Part model, mm, in its own coordinate system. A direction names the side the tool comes from. Give positions to 0.01 mm unless a question says otherwise; leave off trailing zeros. Write each loop counter-clockwise with the first axis right and the second up, starting at its lowest first coordinate (ties: lowest second). Pieces come first, ordered by that corner, then holes. Notation, with made-up numbers: M 23,56 L 70,56 A32 ccw 70,84 Z; hole C 13.25,30.25 d2. An arc over 180 degrees is marked long. Use CSV: the item, a comma, the result in double quotes. Start each with the question number.
1. Band-saw the part on A-A, the plane y = 59.5. List the corners of the cut face in (x, z).
2. Mould opens along Y. For faces 1 (the face through (43, 68, -11.1)), 2 (the face through (30.5, 23, -9)), 3 (the face through (43, 10, -14)) say: pulls with the +Y half, pulls with the -Y half, needs draft (parallel to the pull), parting line crosses it, or undercut.
3. Band-saw the part on B-B, the plane z = -14. Count the separate pieces of the cut face and the enclosed holes in it, then the cut area to 3 significant figures.
4. Drop flat-ended pins along their axis: pin 1 Ø6 at (x, z) = (28, 6) entering from +Y; pin 2 Ø10 at (x, z) = (27, -9.5) entering from -Y; pin 3 Ø2 at (x, z) = (19, -26.5) entering from +Y. Give the stop position or say it passes through.
5. Drill centre lines: line 1 along Z through (x, y) = (26, 18); line 2 along X through (y, z) = (19, -3); line 3 along X through (y, z) = (6, 4). Where is each one in solid material? Low to high. Write a range as from..to.
6. 3-axis set-ups, long thin cutter, end or side, ignore diameter. For faces 4 (the face through (-43, 30, -27)), 5 (the face through (-43, 10, 0)), 6 (the face through (-41.7, 67, 12.7)): which of +Z, -Z, +X, -X, +Y, -Y reach the whole face in a straight line?
from build123d import *

# Parameters (mm, degrees)
SKETCH1_W                       = 96
SKETCH1_H                       = 68
BOSS_EXTRUDE1_DEPTH             = 80
SKETCH2_W                       = 75
SKETCH2_H                       = 64
CUT_EXTRUDE1_DEPTH              = 45
SKETCH3_W                       = 30
SKETCH3_H                       = 32
CUT_EXTRUDE2_DEPTH              = 8
SKETCH9_R                       = 1.8
CUT_EXTRUDE5_DEPTH              = 80.177016867
CHAMFER1_SIZE                   = 10
SKETCH10_R                      = 10
SKETCH10_R_2                    = 3.8
CUT_EXTRUDE7_DEPTH              = 13
CHAMFER2_SIZE                   = 3
CUT_EXTRUDE8_DEPTH              = 25
SKETCH12_R                      = 1.6
SKETCH12_W                      = 4.5
SKETCH12_H                      = 18
CUT_EXTRUDE9_DEPTH              = 70
SKETCH13_W                      = 5.8
SKETCH13_H                      = 3
CUT_EXTRUDE10_DEPTH             = 130.50675658
CUT_EXTRUDE11_DEPTH             = 5
CUT_EXTRUDE11_DIRECTION_2_REACH = 76.061


with BuildPart() as part:
    # Sketch1 → Boss-Extrude1 (new body)
    with BuildSketch(Plane(origin=(0, 0, 0), x_dir=(1, 0, 0), z_dir=(0, 1, 0))):
        Rectangle(SKETCH1_W, SKETCH1_H)
    extrude(amount=BOSS_EXTRUDE1_DEPTH)

    # Sketch2 → Cut-Extrude1 (cut)
    with BuildSketch(Plane(origin=(0, 80, 0), x_dir=(1, 0, 0), z_dir=(0, 1, 0))):
        Rectangle(SKETCH2_W, SKETCH2_H)
    extrude(amount=-CUT_EXTRUDE1_DEPTH, mode=Mode.SUBTRACT)

    # Sketch3 → Cut-Extrude2 (cut)
    with BuildSketch(Plane(origin=(0, 35, 0), x_dir=(1, 0, 0), z_dir=(0, 1, 0))):
        with Locations((11.5, -4)):
            Rectangle(SKETCH3_W, SKETCH3_H)
    extrude(amount=-CUT_EXTRUDE2_DEPTH, mode=Mode.SUBTRACT)

    # Sketch9 → Cut-Extrude5 (cut, through all)
    with BuildSketch(Plane(origin=(0, 27, 0), x_dir=(1, 0, 0), z_dir=(0, 1, 0))):
        with Locations(Location((11.5, -4, 0), (0, 0, 270))):
            Circle(SKETCH9_R)
    extrude(amount=-CUT_EXTRUDE5_DEPTH, mode=Mode.SUBTRACT)

    # Chamfer1
    chamfer1_edges = [part.edges().sort_by_distance(p)[0] for p in [
        (11.5, 27, 2.2),
    ]]
    chamfer(chamfer1_edges, length=CHAMFER1_SIZE)

    # Sketch10 → Cut-Extrude7 (cut)
    with BuildSketch(Plane.XZ):
        with Locations(Location((11.5, 4, 0), (0, 0, 270))):
            Circle(SKETCH10_R)
        with Locations(Location((11.5, 4, 0), (0, 0, 270))):
            Circle(SKETCH10_R_2, mode=Mode.SUBTRACT)
    extrude(amount=-CUT_EXTRUDE7_DEPTH, mode=Mode.SUBTRACT)

    # Chamfer2
    chamfer2_edges = [part.edges().sort_by_distance(p)[0] for p in [
        (11.5, 13, 14),
        (11.5, 13, 7.8),
    ]]
    chamfer(chamfer2_edges, length=CHAMFER2_SIZE)

    # Sketch11 → Cut-Extrude8 (cut)
    with BuildSketch(Plane(origin=(0, 35, 0), x_dir=(1, 0, 0), z_dir=(0, 1, 0))):
        Polygon((9.5, 32), (-37.5, 32), (-37.5, 2), (-7.5, 2), (-7.5, 16), (9.5, 16), align=None)
        Polygon((-7.5, -2), (-37.5, -2), (-37.5, -32), (9.5, -32), (9.5, -24), (-7.5, -24), align=None)
        Polygon((37.5, -32), (37.5, -2), (30.5, -2), (30.5, -24), (13.5, -24), (13.5, -32), align=None)
        Polygon((37.5, 32), (13.5, 32), (13.5, 16), (30.5, 16), (30.5, 2), (37.5, 2), align=None)
    extrude(amount=-CUT_EXTRUDE8_DEPTH, mode=Mode.SUBTRACT)

    # Sketch12 → Cut-Extrude9 (cut)
    with BuildSketch(Plane(origin=(0, 80, 0), x_dir=(1, 0, 0), z_dir=(0, 1, 0))):
        with Locations(Location((-43, 14, 0), (0, 0, 270))):
            Circle(SKETCH12_R)
        with Locations(Location((-43, -14, 0), (0, 0, 90))):
            Circle(SKETCH12_R)
        with Locations(Location((43, -14, 0), (0, 0, 270))):
            Circle(SKETCH12_R)
        with Locations(Location((43, 14, 0), (0, 0, 90))):
            Circle(SKETCH12_R)
        with Locations((-42.75, 0)):
            Rectangle(SKETCH12_W, SKETCH12_H)
        with Locations((42.75, 0)):
            Rectangle(SKETCH12_W, SKETCH12_H)
    extrude(amount=-CUT_EXTRUDE9_DEPTH, mode=Mode.SUBTRACT)

    # Sketch13 → Cut-Extrude10 (cut, through all)
    with BuildSketch(Plane.ZY.offset(48)):
        with Locations((-14, 68.5)):
            Rectangle(SKETCH13_W, SKETCH13_H)
        with Locations((14, 68.5)):
            Rectangle(SKETCH13_W, SKETCH13_H)
    extrude(amount=-CUT_EXTRUDE10_DEPTH, mode=Mode.SUBTRACT)

    # Sketch15 → Cut-Extrude11 (cut)
    with BuildSketch(Plane(origin=(0, 35, 0), x_dir=(1, 0, 0), z_dir=(0, 1, 0))):
        Polygon((-57.5, 28), (-57.5, 21), (39.5, 21), (39.5, 28), (39.5, 32), (-57.5, 32), align=None)
    extrude(amount=-CUT_EXTRUDE11_DEPTH, mode=Mode.SUBTRACT)

    # Cut-Extrude11 direction 2: up to this face of the body (flat: up to its plane)
    cut_extrude11_direction_2_end = Plane(part.part.faces().sort_by_distance((0, 80, -32.823564706))[0])
    # Sketch15 → Cut-Extrude11 direction 2 (cut, up to the picked face)
    with BuildSketch(Plane(origin=(0, 35, 0), x_dir=(1, 0, 0), z_dir=(0, 1, 0)), mode=Mode.PRIVATE) as cut_extrude11_direction_2_sk1:
        Polygon((-57.5, 28), (-57.5, 21), (39.5, 21), (39.5, 28), (39.5, 32), (-57.5, 32), align=None)
    cut_extrude11_direction_2_tool1 = split(extrude(cut_extrude11_direction_2_sk1.sketch, amount=CUT_EXTRUDE11_DIRECTION_2_REACH, mode=Mode.PRIVATE), bisect_by=cut_extrude11_direction_2_end, keep=Keep.BOTH, mode=Mode.PRIVATE)
    add(cut_extrude11_direction_2_tool1.solids().sort_by(Axis((-9, 35, -26.5), (0, 1, 0)))[0], mode=Mode.SUBTRACT)


solid = part.part
Output:
1,outline,"M -48,-34 L 48,-34 L 48,34 L -48,34 L -48,-21 L -37.5,-21 L -37.5,32 L 37.5,32 L 37.5,-21 L 39.5,-21 L 39.5,-32 L -48,-32 Z; hole M -45,-9 L -40.5,-9 L -40.5,9 L -45,9 Z; hole C -43,-14 d3.2; hole C -43,14 d3.2; hole M 40.5,-9 L 45,-9 L 45,9 L 40.5,9 Z; hole C 43,-14 d3.2; hole C 43,14 d3.2"
2,face 1,"undercut"
2,face 2,"needs draft"
2,face 3,"pulls with the +Y half"
3,separate pieces,"5"
3,enclosed holes,"0"
3,area,"2,890 mm²"
4,pin 1,"stops at y = 35"
4,pin 2,"stops at y = 0"
4,pin 3,"stops at y = 10"
5,line 1,"z = -34..-32, -16..24, 32..34"
5,line 2,"x = -48..-45, -40.5..-37.5, -7.5..30.5, 37.5..40.5, 45..48"
5,line 3,"x = -48..1.5, 7.7..9.7, 13.3..15.3, 21.5..48"
6,face 4,"-X, +Y"
6,face 5,"+Y"
6,face 6,"+X, -X"
